from build123d import *

# Parameters (mm, degrees)
BOX469_W               = 8
BOX469_H               = 8
BOX469_DEPTH           = 1
BOX468_W               = 26
BOX468_H               = 13
BOX468_DEPTH           = 1.5
BOX467_W               = 6
BOX467_H               = 7
BOX467_DEPTH           = 3
CYLINDER691_R          = 150
CYLINDER691_DEPTH      = 7
CYLINDER691_ROLL_ANGLE = 90
CYLINDER689_R          = 1.6
CYLINDER689_DEPTH      = 10
CYLINDER690_R          = 1.6
CYLINDER690_DEPTH      = 10
BOX466_W               = 10
BOX466_H               = 10
BOX466_DEPTH           = 10
CYLINDER688_R          = 1.5
CYLINDER688_DEPTH      = 4
CUT576_PLACEMENT_ANGLE = 180
BOX465_W               = 10
BOX465_H               = 10
BOX465_DEPTH           = 10
CYLINDER687_R          = 1.5
CYLINDER687_DEPTH      = 4
CUT575_PLACEMENT_ANGLE = 180
BOX464_W               = 10
BOX464_H               = 10
BOX464_DEPTH           = 10
CYLINDER686_R          = 1.5
CYLINDER686_DEPTH      = 4
BOX463_W               = 10
BOX463_H               = 10
BOX463_DEPTH           = 10
CYLINDER685_R          = 1.5
CYLINDER685_DEPTH      = 4
BOX461_W               = 12
BOX461_H               = 0.5
BOX461_DEPTH           = 1
BOX462_W               = 12
BOX462_H               = 0.5
BOX462_DEPTH           = 1
BOX460_W               = 12
BOX460_H               = 1
BOX460_DEPTH           = 4
BOX459_W               = 12
BOX459_H               = 1
BOX459_DEPTH           = 4
CYLINDER684_R          = 4.5
CYLINDER684_DEPTH      = 4
CYLINDER683_R          = 4.5
CYLINDER683_DEPTH      = 4
BOX458_W               = 12
BOX458_H               = 8
BOX458_DEPTH           = 1


with BuildPart() as box469:
    # Box469 → Box469 (new body)
    with BuildSketch(Plane(origin=(2, -4, 0), x_dir=(1, 0, 0), z_dir=(0, 0, 1))):
        with Locations((4, 4)):
            Rectangle(BOX469_W, BOX469_H)
    extrude(amount=BOX469_DEPTH)


with BuildPart() as box468:
    # Box468 → Box468 (new body)
    with BuildSketch(Plane(origin=(-6, -6, 0), x_dir=(1, 0, 0), z_dir=(0, 0, 1))):
        with Locations((13, 6.5)):
            Rectangle(BOX468_W, BOX468_H)
    extrude(amount=BOX468_DEPTH)


with BuildPart() as box467:
    # Box467 → Box467 (new body)
    with BuildSketch(Plane(origin=(3, -3.5, 1), x_dir=(1, 0, 0), z_dir=(0, 0, 1))):
        with Locations((3, 3.5)):
            Rectangle(BOX467_W, BOX467_H)
    extrude(amount=BOX467_DEPTH)


with BuildPart() as cylinder910:
    # Cylinder691 → Cylinder691 (new body)
    with BuildSketch(Plane.XY):
        Circle(CYLINDER691_R)
    extrude(amount=CYLINDER691_DEPTH)


with BuildPart() as cylinder910_1:
    # Cylinder691 roll: moved
    add(cylinder910.part.rotate(Axis((0, 0, 0), (1, 0, 0)), CYLINDER691_ROLL_ANGLE))


with BuildPart() as cylinder910_2:
    # Cylinder691 placement: moved
    add(cylinder910_1.part.moved(Location((6, 3.5, 153))))


with BuildPart() as cylinder908:
    # Cylinder689 → Cylinder689 (new body)
    with BuildSketch(Plane.XY):
        Circle(CYLINDER689_R)
    extrude(amount=CYLINDER689_DEPTH)


with BuildPart() as fusion458:
    # Cylinder690 → Cylinder690 (new body)
    with BuildSketch(Plane(origin=(12, 0, 0), x_dir=(1, 0, 0), z_dir=(0, 0, 1))):
        Circle(CYLINDER690_R)
    extrude(amount=CYLINDER690_DEPTH)

    # Fusion458: union Cylinder908
    add(cylinder908.part)


with BuildPart() as box466:
    # Box466 → Box466 (new body)
    with BuildSketch(Plane(origin=(-5, 0, 0), x_dir=(1, 0, 0), z_dir=(0, 0, 1))):
        with Locations((5, 5)):
            Rectangle(BOX466_W, BOX466_H)
    extrude(amount=BOX466_DEPTH)


with BuildPart() as cut864:
    # Cylinder688 → Cylinder688 (new body)
    with BuildSketch(Plane.XY):
        Circle(CYLINDER688_R)
    extrude(amount=CYLINDER688_DEPTH)

    # Cut576: cut Box466
    add(box466.part, mode=Mode.SUBTRACT)


with BuildPart() as cut864_1:
    # Cut576 placement: moved
    add(cut864.part.moved(Location((12, 4, 0))).rotate(Axis((12, 4, 0), (0, 0, 1)), CUT576_PLACEMENT_ANGLE))


with BuildPart() as box465:
    # Box465 → Box465 (new body)
    with BuildSketch(Plane(origin=(-5, 0, 0), x_dir=(1, 0, 0), z_dir=(0, 0, 1))):
        with Locations((5, 5)):
            Rectangle(BOX465_W, BOX465_H)
    extrude(amount=BOX465_DEPTH)


with BuildPart() as cut863:
    # Cylinder687 → Cylinder687 (new body)
    with BuildSketch(Plane.XY):
        Circle(CYLINDER687_R)
    extrude(amount=CYLINDER687_DEPTH)

    # Cut575: cut Box465
    add(box465.part, mode=Mode.SUBTRACT)


with BuildPart() as cut863_1:
    # Cut575 placement: moved
    add(cut863.part.moved(Location((0, 4, 0))).rotate(Axis((0, 4, 0), (0, 0, 1)), CUT575_PLACEMENT_ANGLE))


with BuildPart() as box464:
    # Box464 → Box464 (new body)
    with BuildSketch(Plane(origin=(-5, 0, 0), x_dir=(1, 0, 0), z_dir=(0, 0, 1))):
        with Locations((5, 5)):
            Rectangle(BOX464_W, BOX464_H)
    extrude(amount=BOX464_DEPTH)


with BuildPart() as cut862:
    # Cylinder686 → Cylinder686 (new body)
    with BuildSketch(Plane.XY):
        Circle(CYLINDER686_R)
    extrude(amount=CYLINDER686_DEPTH)

    # Cut574: cut Box464
    add(box464.part, mode=Mode.SUBTRACT)


with BuildPart() as cut862_1:
    # Cut574 placement: moved
    add(cut862.part.moved(Location((12, -4, 0))))


with BuildPart() as box463:
    # Box463 → Box463 (new body)
    with BuildSketch(Plane(origin=(-5, 0, 0), x_dir=(1, 0, 0), z_dir=(0, 0, 1))):
        with Locations((5, 5)):
            Rectangle(BOX463_W, BOX463_H)
    extrude(amount=BOX463_DEPTH)


with BuildPart() as cut861:
    # Cylinder685 → Cylinder685 (new body)
    with BuildSketch(Plane.XY):
        Circle(CYLINDER685_R)
    extrude(amount=CYLINDER685_DEPTH)

    # Cut573: cut Box463
    add(box463.part, mode=Mode.SUBTRACT)


with BuildPart() as cut861_1:
    # Cut573 placement: moved
    add(cut861.part.moved(Location((0, -4, 0))))


with BuildPart() as box461:
    # Box461 → Box461 (new body)
    with BuildSketch(Plane(origin=(0, 3.5, 3), x_dir=(1, 0, 0), z_dir=(0, 0, 1))):
        with Locations((6, 0.25)):
            Rectangle(BOX461_W, BOX461_H)
    extrude(amount=BOX461_DEPTH)


with BuildPart() as box462:
    # Box462 → Box462 (new body)
    with BuildSketch(Plane(origin=(0, -4, 3), x_dir=(1, 0, 0), z_dir=(0, 0, 1))):
        with Locations((6, 0.25)):
            Rectangle(BOX462_W, BOX462_H)
    extrude(amount=BOX462_DEPTH)


with BuildPart() as box460:
    # Box460 → Box460 (new body)
    with BuildSketch(Plane(origin=(0, 3, 0), x_dir=(1, 0, 0), z_dir=(0, 0, 1))):
        with Locations((6, 0.5)):
            Rectangle(BOX460_W, BOX460_H)
    extrude(amount=BOX460_DEPTH)


with BuildPart() as box459:
    # Box459 → Box459 (new body)
    with BuildSketch(Plane(origin=(0, -4, 0), x_dir=(1, 0, 0), z_dir=(0, 0, 1))):
        with Locations((6, 0.5)):
            Rectangle(BOX459_W, BOX459_H)
    extrude(amount=BOX459_DEPTH)


with BuildPart() as cylinder801:
    # Cylinder684 → Cylinder684 (new body)
    with BuildSketch(Plane(origin=(12, 0, 0), x_dir=(1, 0, 0), z_dir=(0, 0, 1))):
        Circle(CYLINDER684_R)
    extrude(amount=CYLINDER684_DEPTH)


with BuildPart() as cylinder800:
    # Cylinder683 → Cylinder683 (new body)
    with BuildSketch(Plane.XY):
        Circle(CYLINDER683_R)
    extrude(amount=CYLINDER683_DEPTH)


with BuildPart() as obj1:
    # Box458 → Box458 (new body)
    with BuildSketch(Plane(origin=(0, -4, 0), x_dir=(1, 0, 0), z_dir=(0, 0, 1))):
        with Locations((6, 4)):
            Rectangle(BOX458_W, BOX458_H)
    extrude(amount=BOX458_DEPTH)

    # Fusion454: union Cylinder801, Cylinder800
    add(cylinder801.part)
    add(cylinder800.part)

    # Fusion455: union Box460, Box459
    add(box460.part)
    add(box459.part)

    # Fusion456: union Box461, Box462
    add(box461.part)
    add(box462.part)

    # Fusion457: union Cut864, Cut863, Cut862, Cut861
    add(cut864_1.part)
    add(cut863_1.part)
    add(cut862_1.part)
    add(cut861_1.part)

    # Cut577: cut Fusion458
    add(fusion458.part, mode=Mode.SUBTRACT)

    # Cut578: cut Cylinder910
    add(cylinder910_2.part, mode=Mode.SUBTRACT)

    # Cut579: cut Box467
    add(box467.part, mode=Mode.SUBTRACT)

    # Cut580: cut Box468
    add(box468.part, mode=Mode.SUBTRACT)


with BuildPart() as obj1_1:
    # Cut580 placement: moved
    add(obj1.part.moved(Location((0, 0, -1.5))))

    # Fusion459: union Box469
    add(box469.part)


with BuildPart() as obj1_2:
    # Fusion459 placement: moved
    add(obj1_1.part.moved(Location((92, 124, -42.5))))


solid = obj1_2.part
Input: part model. Units: mm. Frame: model coordinates. A direction names the side the tool comes from. Round coordinates to 2 decimals unless told otherwise and drop trailing zeros. Order: outer loops, then holes, each group sorted by start corner. A loop starts at its lowest first (then second) coordinate and runs counter-clockwise, first axis right, second up. Notation, with made-up numbers: (-11.5, 64) - (-0.5, 64) arc R27 ccw to (-0.5, 83) - close; hole circle Ø9 at (-6.75, 60). An arc over 180 degrees is marked (long way). Answer as a JSON object with one key per item and string values. Group by question number.
(1) Reachability of faces 1 (the face through (98, 128, -41)), 2 (the face through (98, 120, -41)), 3 (the face through (104.7, 125.605, -40.85)) from +Z, -Z, +X, -X, +Y, -Y: full face, straight path, thin tool, end or side. Return the list, or none.
(2) Cut plane B-B (y = 125.25). Return loops of the section in (x, z), then the cut area to 3 significant figures.
(3) Pin query (flat end, axial travel): P1, Ø1.5, axis at x = 102.5, y = 121.5, coming from the +Z side; P2, Ø4, axis at x = 92, y = 124, coming from the +Z side; P3, Ø2.5, axis at x = 104, y = 124, coming from the +Z side; P4, Ø0.6, axis at y = 125.5, z = -41.5, coming from the +X side. Return the tip coordinate at first contact, or that it passes through.
(4) Cut plane A-A (z = -41.7). Return loops of the section in (x, y).
(5) Material intervals for probe 1 along X at (y, z) = (124, -41.2); probe 2 along X at (y, z) = (124, -41.7); probe 3 along X at (y, z) = (125, -41.4), sorted ascending. Write a range as from..to.
(6) Cut plane C-C (x = 96.75). Return loops of the section in (y, z), then the cut area to 3 significant figures.
(7) Cut plane D-D (x = 104). Return loops of the section in (y, z).
(8) Draft query along X for faces 4 (the face through (104, 118.5, -41.3)), 5 (the face through (87.5, 124.1, -41.5)), 6 (the face through (97.9, 120.2, -40)). Return one class per face: released by +X, released by -X, zero draft, split by the parting line, or undercut.
Here are the results:
{
 "1": {"face 1": "+Z, -Z, +Y", "face 2": "+Z, -Z, -Y", "face 3": "+Z"},
 "2": {"outline": "(87.68, -42.5) - (91, -42.5) - (91, -40.84) arc R150 cw to (87.68, -40.64) - close; (93, -42.5) - (103, -42.5) - (103, -40.92) arc R150 cw to (101, -40.97) - (101, -41.5) - (95, -41.5) - (95, -40.97) arc R150 cw to (93, -40.92) - close; (105, -42.5) - (108.32, -42.5) - (108.32, -40.64) arc R150 cw to (105, -40.84) - close", "area": "23.9 mm^2"},
 "3": {"P1": "stops at z = -40.91", "P2": "stops at z = -40.79", "P3": "passes through", "P4": "stops at x = 108.34"},
 "4": {"outline": "(90.52, 119.75) arc R1.5 ccw to (93.48, 119.75) arc R4.5 ccw to (94.06, 120) - (101.94, 120) arc R4.5 ccw to (102.52, 119.75) arc R1.5 ccw to (105.48, 119.75) arc R4.5 ccw to (105.48, 128.25) arc R1.5 ccw to (102.52, 128.25) arc R4.5 ccw to (101.94, 128) - (94.06, 128) arc R4.5 ccw to (93.48, 128.25) arc R1.5 ccw to (90.52, 128.25) arc R4.5 ccw to start; hole circle Ø3.2 at (92, 124); hole circle Ø3.2 at (104, 124)"},
 "5": {"probe 1": "x = 87.5..90.4, 93.6..95, 101..102.4, 105.6..108.5", "probe 2": "x = 87.5..90.4, 93.6..102.4, 105.6..108.5", "probe 3": "x = 87.61..90.75, 93.25..95, 101..102.75, 105.25..108.39"},
 "6": {"outline": "(120, -42.5) - (128, -42.5) - (128, -40) - (127.5, -40) - (127.5, -41.5) - (120.5, -41.5) - (120.5, -40) - (120, -40) - close", "area": "9.50 mm^2"},
 "7": {"outline": "(118.5, -42.5) - (122.4, -42.5) - (122.4, -40.88) - (120.5, -40.88) - (120.5, -40) - (118.5, -40) - close; (125.6, -42.5) - (129.5, -42.5) - (129.5, -40) - (127.5, -40) - (127.5, -40.88) - (125.6, -40.88) - close"},
 "8": {"face 4": "undercut", "face 5": "released by -X", "face 6": "zero draft"}
}
